from build123d import *

# Parameters (mm, degrees)
BOSS_EXTRUDE1_DEPTH = 10
SKETCH2_R           = 2.5
CUT_EXTRUDE1_DEPTH  = 59
BOSS_EXTRUDE2_START = 0.4
SKETCH3_R           = 4
SKETCH3_R_2         = 2.5
BOSS_EXTRUDE2_DEPTH = 0.4


with BuildPart() as part:
    # Sketch1 → Boss-Extrude1 (new body)
    with BuildSketch(Plane(origin=(0, 0, 0), x_dir=(1, 0, 0), z_dir=(0, 1, 0))):
        Polygon((0, -12), (0, -20), (53, -20), (53, 20), (0, 20), (0, 12.4), (45, 12.4), (45, 12), (45, -12), align=None)
    extrude(amount=BOSS_EXTRUDE1_DEPTH)

    # Sketch2 → Cut-Extrude1 (cut)
    with BuildSketch(Plane.XY.offset(20)):
        with Locations((24.27, 5)):
            Circle(SKETCH2_R)
    extrude(amount=-CUT_EXTRUDE1_DEPTH, mode=Mode.SUBTRACT)

    # Sketch3 → Boss-Extrude2 (add)
    with BuildSketch(Plane.XY.offset(-12.4).offset(BOSS_EXTRUDE2_START)):
        with Locations(Location((24.27, 5, 0), (0, 0, 180))):
            Circle(SKETCH3_R)
        with Locations((24.27, 5)):
            Circle(SKETCH3_R_2, mode=Mode.SUBTRACT)
    extrude(amount=-BOSS_EXTRUDE2_DEPTH)


solid = part.part
Part model, mm, in its own coordinate system. A direction names the side the tool comes from. Coordinates: 2 decimals unless noted, no trailing zeros. Loops run counter-clockwise (first coordinate to the right, second up) from the corner with the lowest first, then second, coordinate; pieces in that order, holes last. Notation, with made-up numbers: M 38.5,3.25 L 86.5,3.25 A27 ccw 86.5,39.25 Z; hole C 15.5,-37 d4. An arc over 180 degrees is marked long. Use a Markdown table: item, result. Add a question column.
Q1. Cut at A-A (y = 5). Write the cut outline in (x, z), and give its area (3 significant figures).
Q2. Pin check, flat tips, straight feed: P1, Ø5, axis at y = 4.5, z = 3.5, coming from the -X side; P2, Ø1, axis at y = 8.5, z = -12.5, coming from the -X side; P3, Ø3, axis at x = 11, z = -10.5, coming from the +Y side (1 decimal). Stop position of each tip, or through.
Q3. Probe L1, parallel to Z at x = 37, y = 6.5; L2, parallel to X at y = 4.75, z = 12.5; L3, parallel to Y at x = 24.27, z = 18. List the from-to ranges inside material, lowest first.
Q4. Which spindle directions (+Z, -Z, +X, -X, +Y, -Y) get a long thin tool onto all of the face, cutting with end or side? Do faces 1 (the flat face through (24, 8, -12)), 2 (the flat face through (26, 10, -14)). Say none if no direction does.
Q5. Cut at B-B (x = 34). Write the cut outline in (y, z), and give its area (3 significant figures).
Q6. Mould opens along X. For faces 3 (the flat face through (0, 5, -16)), 4 (the cylindrical face through (28.266, 4.824, -12.197)), 5 (the flat face through (53, 5, 0)), 6 (the flat face through (22.8, 2.7, 12)) say: +X half, -X half, draft (parallel to the pull), parting line (faces both ways), or undercut.
Q7. Cut at C-C (z = -14). Write the cut outline in (x, y), and give its area (3 significant figures).
Q8. Cut at D-D (x = 24.27). Write the cut outline in (y, z), and give its area (3 significant figures).
Worked out:
| question | item | result |
|---|---|---|
| 1 | outline | M 0,-20 L 21.77,-20 L 21.77,-12 L 20.27,-12 L 20.27,-12.4 L 0,-12.4 Z; M 0,12 L 21.77,12 L 21.77,20 L 0,20 Z; M 26.77,-20 L 53,-20 L 53,20 L 26.77,20 L 26.77,12 L 45,12 L 45,-12.4 L 28.27,-12.4 L 28.27,-12 L 26.77,-12 Z |
| 1 | area | 945 mm2 |
| 2 | P1 | stops at x = 45 |
| 2 | P2 | stops at x = 0 |
| 2 | P3 | passes through |
| 3 | L1 | z = -20 to -12.4, 12 to 20 |
| 3 | L2 | x = 0 to 21.78, 26.76 to 53 |
| 3 | L3 | y = 0 to 2.5, 7.5 to 10 |
| 4 | face 1 | -X, +Y, -Y |
| 4 | face 2 | +Z, -Z, +X, -X, +Y |
| 5 | outline | M 0,-20 L 10,-20 L 10,-12.4 L 0,-12.4 Z; M 0,12 L 10,12 L 10,20 L 0,20 Z |
| 5 | area | 156 mm2 |
| 6 | face 3 | -X half |
| 6 | face 4 | undercut |
| 6 | face 5 | +X half |
| 6 | face 6 | draft |
| 7 | outline | M 0,0 L 53,0 L 53,10 L 0,10 Z; hole C 24.27,5 d5 |
| 7 | area | 510 mm2 |
| 8 | outline | M 0,-20 L 2.5,-20 L 2.5,-12 L 1,-12 L 1,-12.4 L 0,-12.4 Z; M 0,12 L 2.5,12 L 2.5,20 L 0,20 Z; M 7.5,-20 L 10,-20 L 10,-12.4 L 9,-12.4 L 9,-12 L 7.5,-12 Z; M 7.5,12 L 10,12 L 10,20 L 7.5,20 Z |
| 8 | area | 79.2 mm2 |
